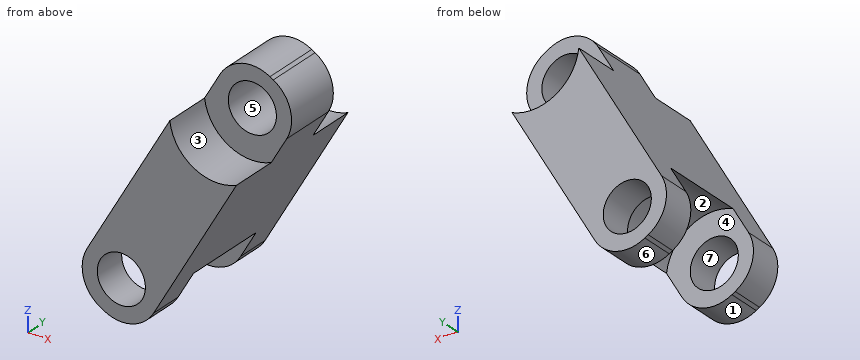
```python
from build123d import *

# Parameters (mm, degrees)
CYLINDER001_R          = 2.5
CYLINDER001_DEPTH      = 2.5
CYLINDER001_ROLL_ANGLE = 90
CYLINDER002_R          = 2.5
CYLINDER002_DEPTH      = 2.5
CYLINDER002_ROLL_ANGLE = 90
CYLINDER_R             = 2.5
CYLINDER_DEPTH         = 4.5
CYLINDER_ROLL_ANGLE    = 90
SKETCH_R               = 1.25
PAD001_DEPTH           = 4
CUT001_PITCH_ANGLE     = -60.000022


with BuildPart() as cylinder001:
    # Cylinder001 → Cylinder001 (new body)
    with BuildSketch(Plane.XY):
        Circle(CYLINDER001_R)
    extrude(amount=CYLINDER001_DEPTH)


with BuildPart() as cylinder001_1:
    # Cylinder001 roll: moved
    add(cylinder001.part.rotate(Axis((0, 0, 0), (1, 0, 0)), CYLINDER001_ROLL_ANGLE))


with BuildPart() as cylinder001_2:
    # Cylinder001 placement: moved
    add(cylinder001_1.part.moved(Location((5, 4, 0))))


with BuildPart() as cylinder002:
    # Cylinder002 → Cylinder002 (new body)
    with BuildSketch(Plane.XY):
        Circle(CYLINDER002_R)
    extrude(amount=CYLINDER002_DEPTH)


with BuildPart() as cylinder002_1:
    # Cylinder002 roll: moved
    add(cylinder002.part.rotate(Axis((0, 0, 0), (1, 0, 0)), CYLINDER002_ROLL_ANGLE))


with BuildPart() as cylinder002_2:
    # Cylinder002 placement: moved
    add(cylinder002_1.part.moved(Location((5, -1.5, 0))))


with BuildPart() as axes_cutout001:
    # Cylinder → Cylinder (new body)
    with BuildSketch(Plane.XY):
        Circle(CYLINDER_R)
    extrude(amount=CYLINDER_DEPTH)


with BuildPart() as axes_cutout001_1:
    # Cylinder roll: moved
    add(axes_cutout001.part.rotate(Axis((0, 0, 0), (1, 0, 0)), CYLINDER_ROLL_ANGLE))


with BuildPart() as axes_cutout001_2:
    # Cylinder placement: moved
    add(axes_cutout001_1.part.moved(Location((-5, 2.25, 0))))

    # Fusion001: union Cylinder001, Cylinder002
    add(cylinder001_2.part)
    add(cylinder002_2.part)


with BuildPart() as track_shape001:
    # Sketch → Pad001 (new body, symmetric)
    with BuildSketch(Plane.XZ):
        with BuildLine():
            Line((-5.1, 2), (5.1, 2))
            ThreePointArc((7, 0.1), (6.443503, 1.443503), (5.1, 2))
            Line((7, 0.1), (7, -0.1))
            ThreePointArc((5.1, -2), (6.443503, -1.443503), (7, -0.1))
            Line((5.1, -2), (-5.1, -2))
            ThreePointArc((-7, -0.1), (-6.443503, -1.443503), (-5.1, -2))
            Line((-7, -0.1), (-7, 0.1))
            ThreePointArc((-5.1, 2), (-6.443503, 1.443503), (-7, 0.1))
        make_face()
        with Locations((-5, 0)):
            Circle(SKETCH_R, mode=Mode.SUBTRACT)
        with Locations((5, 0)):
            Circle(SKETCH_R, mode=Mode.SUBTRACT)
    extrude(amount=PAD001_DEPTH, both=True)

    # Cut001: cut axes-cutout001
    add(axes_cutout001_2.part, mode=Mode.SUBTRACT)


with BuildPart() as track_shape001_1:
    # Cut001 pitch: moved
    add(track_shape001.part.rotate(Axis((0, 0, 0), (0, 1, 0)), CUT001_PITCH_ANGLE))


with BuildPart() as track_shape001_2:
    # Cut001 placement: moved
    add(track_shape001_1.part.moved(Location((7.47807, 0.000117, 4.333453))))


solid = track_shape001_2.part
```
For this review, take the finished solid that the model builds, in its own axes (mm). Face numbers are marked on the shaded views. A direction names the side the tool comes from. Round coordinates to 2 decimals unless told otherwise and drop trailing zeros. Loops run counter-clockwise (first coordinate to the right, second up) from the corner with the lowest first, then second, coordinate; pieces in that order, holes last.
(1) We need section D-D (y = -0.75). Give the boundary of the cut face in (x, z).
Returned:
outline: (4, 2.3) arc R2.5 cw to (7.46, 0.3) - (11.76, 7.75) arc R1.9 ccw to (11.06, 10.35) - (10.89, 10.45) arc R1.9 ccw to (8.3, 9.75) - close; hole circle Ø2.5 at (9.98, 8.66)
(2) Clearance check with flat-ended pins moving along their axes: P1, Ø2, axis at x = 4.98, z = 0, coming from the +Y side; P2, Ø2.5, axis at x = 9.5, z = 8, coming from the -Y side; P3, Ø1, axis at x = 10.5, y = -3, coming from the -Z side. State where each tip first meets the part, or that it passes through.
Returned:
P1: passes through
P2: stops at y = -1.5
P3: stops at z = 4.7
(3) We need section A-A (x = 9). Give the boundary of the cut face in (y, z).
Returned:
outline: (-4, 2.97) - (4, 2.97) - (4, 6.36) - (1.5, 6.36) - (1.5, 7.89) - (-1.5, 7.89) - (-1.5, 6.36) - (-4, 6.36) - close; (-1.5, 9.44) - (1.5, 9.44) - (1.5, 10.45) - (-1.5, 10.45) - close
(4) Tool access review of the marked faces 1, 2 and 3: name each direction out of +Z, -Z, +X, -X, +Y, -Y from which nothing blocks a thin tool from reaching the whole face with its end or side.
Returned:
face 1: -Z, +Y, -Y
face 2: -Z
face 3: +Z, -Y
(5) Mouldability with a two-part tool opening along Z and no side actions: class the marked faces 4, 5, 6 and 7 as released by +Z, released by -Z, zero draft, split by the parting line, or undercut.
Returned:
face 4: zero draft
face 5: undercut
face 6: released by -Z
face 7: undercut
(6) Wall thickness on line 1 along Z through (x, y) = (10, 0); line 2 along Y through (x, z) = (8.5, 8.5); line 3 along Z through (x, y) = (9.25, -1.25): over which ranges is each line inside the solid? List them lowest first.
Returned:
line 1: z = 4.7 to 7.41, 9.91 to 10.7
line 2: y = -1.5 to 1.5
line 3: z = 3.4 to 7.65, 9.68 to 10.57
(7) We need section B-B (z = 0.75). Give the boundary of the cut face in (x, y), plus the area to 3 significant figures.
Returned:
outline: (3.11, -4) - (3.98, -4) - (3.98, -2.25) - (3.11, -2.25) - close; (3.11, 2.25) - (3.98, 2.25) - (3.98, 4) - (3.11, 4) - close; (5.98, -4) - (7.72, -4) - (7.72, 4) - (5.98, 4) - (5.98, 2.25) - (7.36, 2.25) - (7.36, -2.25) - (5.98, -2.25) - close
area: 10.7 mm2
(8) We need section C-C (z = 9.25). Give the boundary of the cut face in (x, y).
Returned:
outline: (8.01, -1.5) - (8.87, -1.5) - (8.87, 1.5) - (8.01, 1.5) - close; (11.08, -1.5) - (11.93, -1.5) - (11.93, 1.5) - (11.08, 1.5) - close
